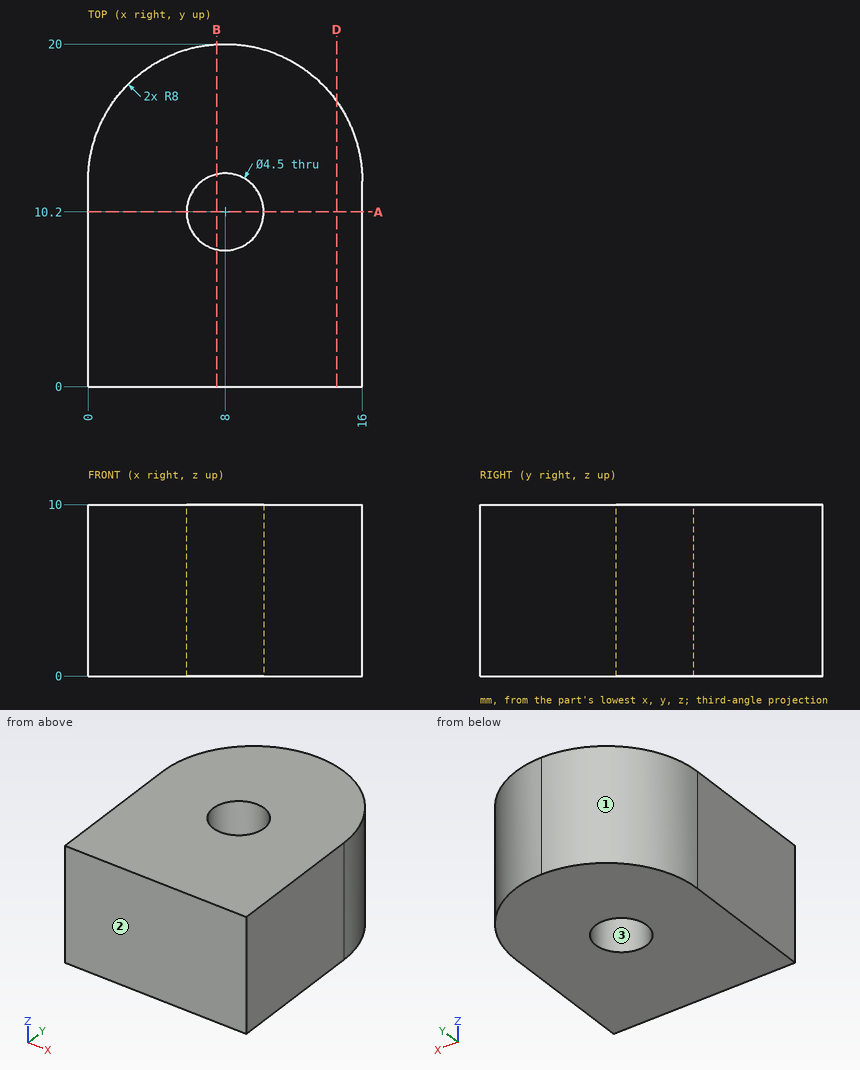
Job drawing, mm, ordinate dimensions from the low corner. One solid piece. Give positions to 0.01 mm unless a question says otherwise; leave off trailing zeros. Write each loop counter-clockwise with the first axis right and the second up, starting at its lowest first coordinate (ties: lowest second). Pieces come first, ordered by that corner, then holes. Notation, with made-up numbers: M 62.5,88 L 117.5,88 A25 cw 117.5,105 Z; hole C 65,55 d8. An arc over 180 degrees is marked long. One line per item, written item: value. Start each with the question number.
Q1. Saw through at D-D, the plane x = 14.5. Write the cut outline in (y, z).
Q2. Saw through at B-B, the plane x = 7.5. Write the cut outline in (y, z), plus the area to 3 significant figures.
Q3. Two-plate mould, pull along X, no slides. Class the marked faces 1, 2 and 3: +X half, -X half, draft (parallel to the pull), parting line (faces both ways), or undercut.
Q4. Probe probe 1 along Y at (x, z) = (8, 2.75); probe 2 along Y at (x, z) = (10, 7.25) (1 decimal); probe 3 along X at (y, z) = (9, 9.75). List the from-to ranges inside material, lowest first. Write a range as [from, to].
Q5. Saw through at A-A, the plane y = 10.2. Write the cut outline in (x, z).
Q6. Drop flat-ended pins along their axis: pin 1 Ø6 at (x, z) = (3, 9) entering from +Y; pin 2 Ø1.5 at (y, z) = (16.5, 2.5) entering from -X. Give the stop position or say it passes through.
Output values:
1. outline: M 0,0 L 16.66,0 L 16.66,10 L 0,10 Z
2. outline: M 0,0 L 8.01,0 L 8.01,10 L 0,10 Z; M 12.39,0 L 19.98,0 L 19.98,10 L 12.39,10 Z
2. area: 156 mm²
3. face 1: -X half
3. face 2: draft
3. face 3: undercut
4. probe 1: y = [0, 7.95], [12.45, 20]
4. probe 2: y = [0, 9.2], [11.2, 19.7]
4. probe 3: x = [0, 6.1], [9.9, 16]
5. outline: M 0,0 L 5.75,0 L 5.75,10 L 0,10 Z; M 10.25,0 L 16,0 L 16,10 L 10.25,10 Z
6. pin 1: stops at y = 19.75
6. pin 2: stops at x = 0.93
